from build123d import *

# Parameters (mm, degrees)
SKETCH1_W                                  = 410.21
SKETCH1_H                                  = 173.99
EXTRUDE1_DEPTH                             = 38.1
EXTRUDE2_DEPTH                             = 0.762
F_3_8_16_TAPPED_HOLE2_AT_2_COUNT           = 2
F_3_8_16_TAPPED_HOLE2_AT_2_PITCH           = 148.59
F_3_8_16_TAPPED_HOLE2_AT_3_COUNT           = 2
F_3_8_16_TAPPED_HOLE2_AT_3_PITCH           = 412.501786905
F_3_8_16_TAPPED_HOLE2_AT_4_COUNT           = 2
F_3_8_16_TAPPED_HOLE2_AT_4_PITCH           = 384.81
FILLET1_R                                  = 10.16
F_3_8_DOWEL_PIN_HOLE_D                     = 9.54278
F_3_8_DOWEL_PIN_HOLE_DEPTH                 = 19.05
F_3_8_DOWEL_PIN_HOLE_CSINK_D               = 14.224
F_3_8_DOWEL_PIN_HOLE_CSINK_ANGLE           = 90
F_3_8_DOWEL_PIN_HOLE_TIP                   = 4.77139
EXTRUDE3_DEPTH                             = 19.05
CHAMFER1_SIZE                              = 2.286
F_7_32_0_21875_DIAMETER_HOLE_VENTED_HOLE_D = 7.14375


with BuildPart() as part:
    # Sketch1 → Extrude1 (new body, symmetric)
    with BuildSketch(Plane(origin=(0, 0, 0), x_dir=(1, 0, 0), z_dir=(0, 1, 0))):
        Rectangle(SKETCH1_W, SKETCH1_H)
    extrude(amount=EXTRUDE1_DEPTH, both=True)

    # Sketch2 → Extrude2 (cut)
    with BuildSketch(Plane(origin=(0, 38.1, 0), x_dir=(1, 0, 0), z_dir=(0, 1, 0))):
        Polygon((-205.105, 61.595), (-179.705, 61.595), (-179.705, 86.995), (179.705, 86.995), (179.705, 61.595), (205.105, 61.595), (205.105, -61.595), (179.705, -61.595), (179.705, -86.995), (-179.705, -86.995), (-179.705, -61.595), (-205.105, -61.595), align=None)
    extrude(amount=-EXTRUDE2_DEPTH, mode=Mode.SUBTRACT)

    # Sketch3 → 3/8-16 Tapped Hole2 (revolve, cut)
    with BuildSketch(Plane(origin=(-192.405, 38.1, -74.295), x_dir=(0, 0, 1), z_dir=(1, 0, 0))):
        Polygon((0, 0), (0, 76.2), (3.96875, 76.2), (3.96875, 25.4), (4.7625, 25.4), (4.7625, 0.366617421), (5.3975, 0), align=None)
    f_3_8_16_tapped_hole2 = revolve(axis=Axis((-192.405, 44.45, -74.295), (0, -1, 0)), mode=Mode.SUBTRACT)

    # 3/8-16 Tapped Hole2 at 2: 3/8-16 Tapped Hole2 ×2
    with Locations(*[(0, 0, i * F_3_8_16_TAPPED_HOLE2_AT_2_PITCH) for i in range(1, F_3_8_16_TAPPED_HOLE2_AT_2_COUNT)]):
        add(f_3_8_16_tapped_hole2, mode=Mode.SUBTRACT)

    # 3/8-16 Tapped Hole2 at 3: 3/8-16 Tapped Hole2 ×2
    with Locations(*[Vector(0.932868686, 0, 0.360216621) * (i * F_3_8_16_TAPPED_HOLE2_AT_3_PITCH) for i in range(1, F_3_8_16_TAPPED_HOLE2_AT_3_COUNT)]):
        add(f_3_8_16_tapped_hole2, mode=Mode.SUBTRACT)

    # 3/8-16 Tapped Hole2 at 4: 3/8-16 Tapped Hole2 ×2
    with Locations(*[(i * F_3_8_16_TAPPED_HOLE2_AT_4_PITCH, 0, 0) for i in range(1, F_3_8_16_TAPPED_HOLE2_AT_4_COUNT)]):
        add(f_3_8_16_tapped_hole2, mode=Mode.SUBTRACT)

    # Fillet1
    fillet1_edges = [part.edges().sort_by_distance(p)[0] for p in [
        (-205.105, 0, -86.995),
        (205.105, 0, -86.995),
        (205.105, 0, 86.995),
        (-205.105, 0, 86.995),
    ]]
    fillet(fillet1_edges, radius=FILLET1_R)

    # 3/8 dowel pin hole
    with Locations(Plane(origin=(0, 37.338, 0), x_dir=(-1, 0, 0), z_dir=(0, 1, 0))):
        with Locations((186.055, 0)):
            CounterSinkHole(F_3_8_DOWEL_PIN_HOLE_D / 2, F_3_8_DOWEL_PIN_HOLE_CSINK_D / 2, depth=F_3_8_DOWEL_PIN_HOLE_DEPTH, counter_sink_angle=F_3_8_DOWEL_PIN_HOLE_CSINK_ANGLE)
            with Locations((0, 0, -(F_3_8_DOWEL_PIN_HOLE_DEPTH + F_3_8_DOWEL_PIN_HOLE_TIP / 2))):  # 90° drill point
                Cone(0, F_3_8_DOWEL_PIN_HOLE_D / 2, F_3_8_DOWEL_PIN_HOLE_TIP, mode=Mode.SUBTRACT)

    # Sketch7 → Extrude3 (cut)
    with BuildSketch(Plane(origin=(0, 37.338, 0), x_dir=(1, 0, 0), z_dir=(0, 1, 0))):
        with BuildLine():
            Line((183.515, 4.77139), (188.595, 4.77139))
            ThreePointArc((188.595, 4.77139), (193.36639, 0), (188.595, -4.77139))
            Line((188.595, -4.77139), (183.515, -4.77139))
            ThreePointArc((183.515, -4.77139), (178.74361, 0), (183.515, 4.77139))
        make_face()
    extrude(amount=-EXTRUDE3_DEPTH, mode=Mode.SUBTRACT)

    # Chamfer1
    chamfer1_edges = [part.edges().sort_by_distance(p)[0] for p in [
        (178.74361, 37.338, 0),
        (186.055, 37.338, 4.77139),
        (193.36639, 37.338, 0),
        (186.055, 37.338, -4.77139),
    ]]
    chamfer(chamfer1_edges, length=CHAMFER1_SIZE)

    # 7/32 (0.21875) Diameter Hole Vented Holes (through all)
    with Locations(Plane(origin=(0, 37.338, 0), x_dir=(-1, 0, 0), z_dir=(0, 1, 0))):
        with Locations((-186.055, 0), (186.055, 0)):
            Hole(F_7_32_0_21875_DIAMETER_HOLE_VENTED_HOLE_D / 2)


solid = part.part
Here's how the part is built. I have some questions about the finished solid (model axes, mm). A direction names the side the tool comes from. Give positions to 0.01 mm unless a question says otherwise; leave off trailing zeros. Answer as a JSON object with one key per item and string values. Group by question number.
1) On a 3-axis mill with a long thin cutter (end or side, diameter ignored), from which of +Z, -Z, +X, -X, +Y, -Y can I reach the whole of each face in a straight line? I mean faces 1 (the flat face through (189, 12.7, 77)), 2 (the flat face through (-205.105, 1, 1)). Say none if no direction works.
2) Please list where these lines run through material, in increasing order: L1, parallel to X at y = -28.5, z = 75 (3 decimals); L2, parallel to X at y = -30, z = 72.5 (3 decimals); L3, parallel to Y at x = -184, z = 39. Write a range as [from, to].
3) I'm going to push flat-ended pins straight in: pin 1 Ø0.8 at (y, z) = (38, -79) entering from +X; pin 2 Ø7.5 at (x, z) = (-186.055, 0) entering from +Y; pin 3 Ø7.5 at (x, z) = (185.5, 1.5) entering from +Y; pin 4 Ø3 at (x, z) = (193, 76) entering from +Y. Where does each tip first touch, or does it pass through?
4) We'd pull the mould along Z, two halves only. Please class faces 3 (the cylindrical face through (189.72, -12.34, 71.37)), 4 (the flat face through (-3, -38.1, -1)), 5 (the cylindrical face through (202.05, 0.53, 84.1)): pulls with the +Z half, pulls with the -Z half, needs draft (parallel to the pull), parting line crosses it, or undercut.
Results found:
{
 "1": {"face 1": "+Y", "face 2": "+Z, -Z, -X, +Y, -Y"},
 "2": {"L1": "[-205.105, -196.311], [-188.499, 188.499], [196.311, 205.105]", "L2": "[-205.105, -195.945], [-188.865, 188.865], [195.945, 205.105]", "L3": "[-38.1, 37.34]"},
 "3": {"pin 1": "x = 204.95", "pin 2": "y = 17.27", "pin 3": "y = 35.53", "pin 4": "through"},
 "4": {"face 3": "undercut", "face 4": "needs draft", "face 5": "pulls with the +Z half"}
}
